Can you work these out from the model? Positions are in its coordinate system, mm. Face numbers are marked on the shaded views. A direction names the side the tool comes from. Round coordinates to 2 decimals unless told otherwise and drop trailing zeros. Order: outer loops, then holes, each group sorted by start corner. A loop starts at its lowest first (then second) coordinate and runs counter-clockwise, first axis right, second up. Notation, with made-up numbers: M 84,-18 L 98,-18 A23 cw 98,19 Z; hole C 67.5,-18 d4. An arc over 180 degrees is marked long. Answer as a JSON object with one key per item and string values. Group by question number.
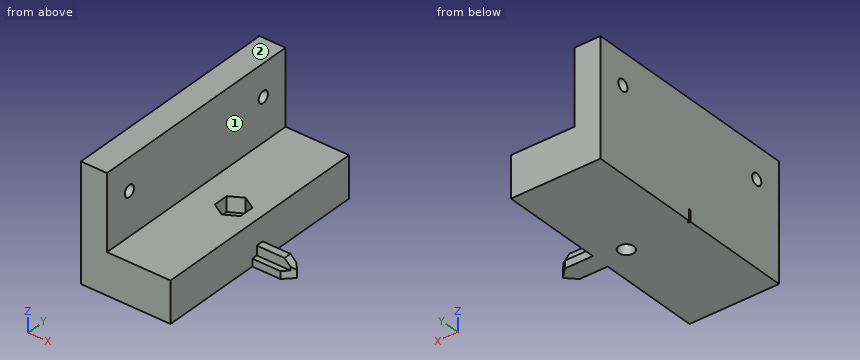
Autodesk Inventor part; units mm, degrees
ref_plane "YZ Plane" through (0, 0, 0) normal (1, 0, 0) x (0, 1, 0)
ref_plane "XZ Plane" through (0, 0, 0) normal (0, 1, 0) x (-1, 0, 0)
ref_plane "XY Plane" through (0, 0, 0) normal (0, 0, 1) x (1, 0, 0)
sketch "Skizze1" plane through (0, 0, 0) normal (0, 0, 1) x (1, 0, 0)
  line L0 (-13.5, 30) -> (13.5, 30)
  line L1 (13.5, 30) -> (13.5, -30)
  line L2 (13.5, -30) -> (-13.5, -30)
  line L3 (-13.5, -30) -> (-13.5, 30)
  line L4 (-13.5, 30) -> (13.5, -30) construction
  line L5 (13.5, 30) -> (-13.5, -30) construction
  point P0 (0, 0)
  dimension "d0" = 27
  dimension "d1" = 60
extrude "Extrusion1" add sketch "Skizze1" along normal blind 11
sketch "Skizze2" plane through (0, 0, 11) normal (0, 0, 1) x (1, 0, 0)
  line L0 (13.5, 30) -> (-13.5, 30)
  line L1 (-13.5, -30) -> (13.5, -30)
  line L2 (-13.5, 30) -> (-3.5, 30)
  line L3 (-3.5, 30) -> (-3.5, -30)
  line L4 (-3.5, -30) -> (-13.5, -30)
  line L5 (-13.5, -30) -> (-13.5, 30)
  point P0 (0, 0)
  dimension "d4" = 10
extrude "Extrusion2" add sketch "Skizze2" along normal blind 20
sketch "Skizze3" plane through (-3.5, -30, 11) normal (1, 0, 0) x (0, 0, -1)
  line L0 (0, 60) -> (0, 0) construction
  line L1 (0, 60) -> (-20, 60) construction
  line L2 (-20, 0) -> (-20, 60) construction
  line L3 (0, 0) -> (-20, 0) construction
  line L4 (0, 60) -> (0, 0)
  line L5 (0, 30) -> (-11.5, 30) construction
  line L6 (-11.5, 30) -> (-11.5, 52.5) construction
  line L7 (-11.5, 30) -> (-11.5, 7.5) construction
  circle A0 centre (-11.5, 7.5) radius 1.55
  circle A1 centre (-11.5, 52.5) radius 1.55
  point P0 (11, 30)
  dimension "d7" = 11.5
  dimension "d8" = 22.5
  dimension "d9" = 22.5
  dimension "d10" = 3.1
  dimension "d11" = 3.1
extrude "Extrusion3" cut sketch "Skizze3" against normal through all
sketch "Skizze4" plane through (-13.5, -30, 0) normal (-1, 0, 0) x (0, 0, 1)
  circle A0 centre (22.5, 7.5) radius 1.55
  circle A1 centre (22.5, 52.5) radius 1.55
  line L0 (0, 0) -> (0, 60)
  line L1 (0, 0) -> (31, 0)
  line L2 (31, 60) -> (31, 0)
  line L3 (0, 60) -> (31, 60)
  point P0 (0, 30)
extrude "Extrusion4" cut sketch "Skizze4" against normal blind 3
sketch "Skizze5" plane through (-10.5, -30, 0) normal (-1, 0, 0) x (0, 0, 1)
  line L0 (-3, 30.25) -> (3, 30.25)
  line L1 (3, 30.25) -> (3, 29.75)
  line L2 (3, 29.75) -> (-3, 29.75)
  line L3 (-3, 29.75) -> (-3, 30.25)
  line L4 (-3, 30.25) -> (3, 29.75) construction
  line L5 (3, 30.25) -> (-3, 29.75) construction
  point P0 (0, 30)
  dimension "d16" = 6
  dimension "d17" = 0.5
extrude "Extrusion5" cut sketch "Skizze5" against normal blind 0.5
sketch "Skizze6" plane through (0, 0, 11) normal (0, 0, 1) x (1, 0, 0)
  line L0 (-3.5, -30) -> (-3.5, 30)
  line L1 (-3.5, 0) -> (6.5, 0)
  circle A0 centre (6.5, 0) radius 2.05
  point P0 (0, 0)
  dimension "d20" = 10
  dimension "d21" = 4.1
extrude "Extrusion6" cut sketch "Skizze6" against normal through all
sketch "Skizze7" plane through (0, 0, 11) normal (0, 0, 1) x (1, 0, 0)
  circle A0 centre (6.5, 0) radius 2.05
  line L0 (6.5, 0) -> (6.5, 4)
  line L1 (6.5, 0) -> (14.5, 0) construction
  line L2 (6.5, 4) -> (9.9641, 2)
  line L3 (9.9641, 2) -> (9.9641, -2)
  line L4 (9.9641, -2) -> (6.5, -4)
  line L5 (6.5, -4) -> (3.0359, -2)
  line L6 (3.0359, -2) -> (3.0359, 2)
  line L7 (3.0359, 2) -> (6.5, 4)
  point P0 (0, 0)
  dimension "d24" = 4
extrude "Extrusion7" cut sketch "Skizze7" against normal blind 4
sketch "Skizze8" plane through (13.5, -30, 0) normal (1, 0, 0) x (0, 0, -1)
  line L0 (0, 27.5) -> (-2, 27.5)
  line L1 (-2, 32.5) -> (0, 32.5)
  line L2 (2, 27.5) -> (-2, 32.5) construction
  line L3 (-2, 27.5) -> (2, 32.5) construction
  line L4 (0, 27.5) -> (0, 32.5)
  line L5 (0, 30.25) -> (0, 60)
  line L6 (-4.5, 29) -> (-4.5, 31)
  line L7 (-4.5, 31) -> (-2, 31)
  line L8 (0, 29.2) -> (-4.5, 31) construction
  line L9 (-4.5, 29) -> (0, 30.8) construction
  line L10 (-2, 27.5) -> (-2, 29)
  line L11 (-2, 31) -> (-2, 32.5)
  line L12 (-2, 29) -> (-4.5, 29)
  point P0 (0, 30)
extrude "Extrusion8" add sketch "Skizze8" along normal blind 10
sketch "Skizze9" plane through (13.5, -1, 4.5) normal (0, 0, 1) x (1, 0, 0)
  line L0 (10, -1.5) -> (10, 3.5)
  line L1 (10, 1) -> (7.5, -1.5)
  line L2 (0, -1.5) -> (10, -1.5)
  line L3 (10, 1) -> (13.5355, 1) construction
  line L4 (7.5, -1.5) -> (10, -1.5)
  line L5 (0, 3.5) -> (10, 3.5)
  line L6 (10, -1.5) -> (10, 3.5)
  line L7 (10, 3.5) -> (7.5, 3.5)
  line L8 (10, 1) -> (7.5, 3.5)
  point P0 (-13.5, 1)
  dimension "d35" = 135
extrude "Extrusion9" cut sketch "Skizze9" against normal blind 10
sketch "Skizze10" plane through (13.5, -2.5, 0) normal (0, -1, 0) x (1, 0, 0)
  line L0 (10, 4.5) -> (9, 4.5)
  line L1 (10, 4.5) -> (10, 1.9816)
  line L2 (10, 0) -> (10, 4.5)
  line L3 (10, 1.9816) -> (7.4258, 4.5)
  line L4 (0, 4.5) -> (9, 4.5)
  line L5 (10, 4.5) -> (7.4258, 4.5)
  point P0 (-13.5, 0)
extrude "Extrusion10" cut sketch "Skizze10" against normal blind 10
properties part number "cam_holder_hog_part"
Item 1: I'm going to push flat-ended pins straight in: pin 1 Ø5 at (x, y) = (8.5, 15) entering from +Z; pin 2 Ø2 at (y, z) = (3.5, 24.5) entering from +X; pin 3 Ø0.8 at (x, z) = (17, 3.5) entering from -Y. Where does each tip first touch, or does it pass through?
Item 2: Suppose I cut it at A-A, the plane z = 9. Write out the boundary of the cut face in (x, y).
Item 3: Suppose I cut it at B-B, the plane y = 22.5. Write out the boundary of the cut face in (x, z), and give its area (3 significant figures).
Item 4: Suppose I cut it at D-D, the plane y = -18. Write out the boundary of the cut face in (x, z), and give its area (3 significant figures).
Item 5: On a 3-axis mill with a long thin cutter (end or side, diameter ignored), from which of +Z, -Z, +X, -X, +Y, -Y can I reach the whole of each face in a straight line? I mean the marked faces 1 and 2. Say none if no direction works.
Item 6: I need wall thicknesses on line 1 (Y direction, x = -8, z = 22.5); line 2 (X direction, y = 23.5, z = 18); line 3 (Z direction, x = -5, y = -22). Which ranges of each line are inside material? Lowest first, please.
Item 7: Suppose I cut it at C-C, the plane z = 22.5. Write out the boundary of the cut face in (x, y).
Computed:
{
 "1": {"pin 1": "stops at z = 11", "pin 2": "stops at x = -3.5", "pin 3": "stops at y = -1"},
 "2": {"outline": "M -10.5,-30 L 13.5,-30 L 13.5,30 L -10.5,30 Z; hole M 3.04,-2 L 6.5,-4 L 9.96,-2 L 9.96,2 L 6.5,4 L 3.04,2 Z"},
 "3": {"outline": "M -10.5,0 L 13.5,0 L 13.5,11 L -3.5,11 L -3.5,20.95 L -10.5,20.95 Z; M -10.5,24.05 L -3.5,24.05 L -3.5,31 L -10.5,31 Z", "area": "382 mm^2"},
 "4": {"outline": "M -10.5,0 L 13.5,0 L 13.5,11 L -3.5,11 L -3.5,31 L -10.5,31 Z", "area": "404 mm^2"},
 "5": {"face 1": "+Z, +X, +Y, -Y", "face 2": "+Z, +X, -X, +Y, -Y"},
 "6": {"line 1": "y = -30 to -24.05, -20.95 to 20.95, 24.05 to 30", "line 2": "x = -10.5 to -3.5", "line 3": "z = 0 to 21.03, 23.97 to 31"},
 "7": {"outline": "M -10.5,-30 L -3.5,-30 L -3.5,-24.05 L -10.5,-24.05 Z; M -10.5,-20.95 L -3.5,-20.95 L -3.5,20.95 L -10.5,20.95 Z; M -10.5,24.05 L -3.5,24.05 L -3.5,30 L -10.5,30 Z"}
}
